The figure shows three views and two pictorial views of one solid part (mm, origin at its lowest corner). Answer the questions. Coordinates: 2 decimals unless noted, no trailing zeros. Order: outer loops, then holes, each group sorted by start corner. A loop starts at its lowest first (then second) coordinate and runs counter-clockwise, first axis right, second up.
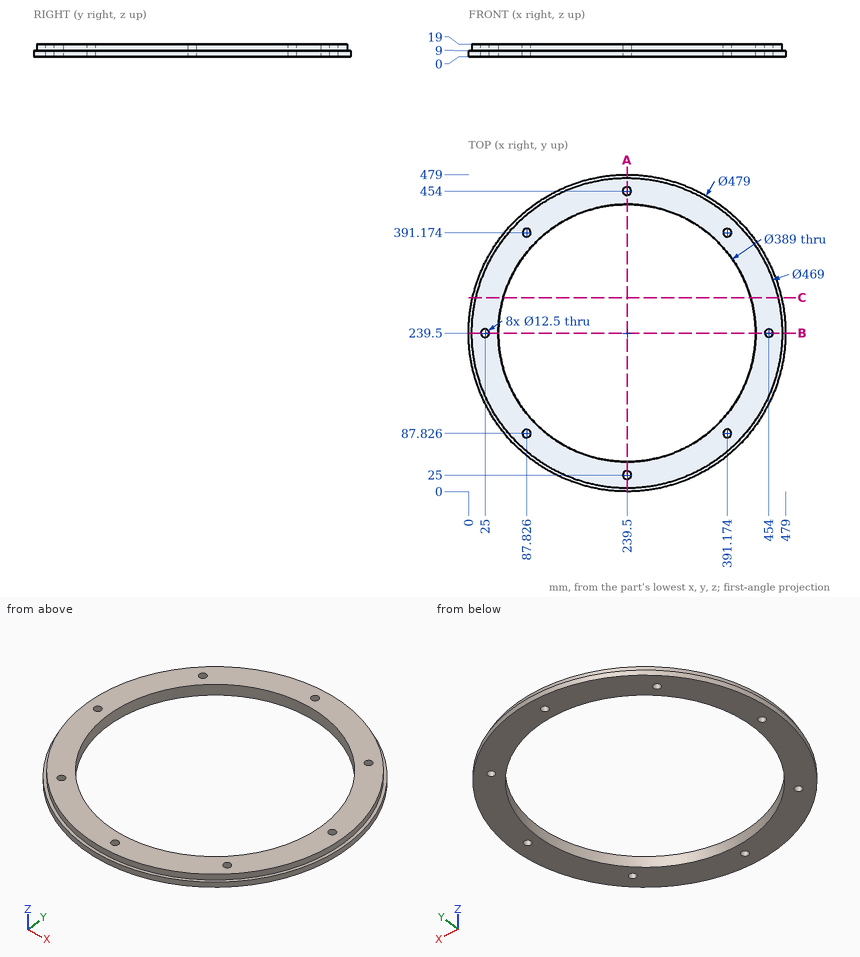
Q1. The part is cut by section C-C, the plane y = 293. Determine the outline of the cut face in (x, z) (1 decimal).
Q2. The part is cut by section A-A, the plane x = 239.5. Determine the outline of the cut face in (y, z), then the cut area to 4 significant figures.
Q3. Each of these flat-tipped pins is pushed along its axis until it touches: P1, Ø5, axis at y = 311, z = 5, coming from the -X side (1 decimal); P2, Ø10, axis at y = 112, z = 2.5, coming from the -X side; P3, Ø3, axis at x = 419, z = 5, coming from the +Y side. Where does it stop, or does it pass through?
Q4. Straight lines are drawn through the part: L1, parallel to Y at x = 239.5, z = 11.5; L2, parallel to Y at x = 239.5, z = 4.75; L3, parallel to X at y = 88.5, z = 13.25 (1 decimal). For each, find the intervals that lie inside material, in ascending order.
Computed values:
1. outline: (6.1, 0) - (52.5, 0) - (52.5, 19) - (11.2, 19) - (11.2, 9) - (6.1, 9) - close; (426.5, 0) - (472.9, 0) - (472.9, 9) - (467.8, 9) - (467.8, 19) - (426.5, 19) - close
2. outline: (0, 0) - (18.75, 0) - (18.75, 19) - (5, 19) - (5, 9) - (0, 9) - close; (31.25, 0) - (45, 0) - (45, 19) - (31.25, 19) - close; (434, 0) - (447.75, 0) - (447.75, 19) - (434, 19) - close; (460.25, 0) - (479, 0) - (479, 9) - (474, 9) - (474, 19) - (460.25, 19) - close
2. area: 1,135 mm2
3. P1: stops at x = 10.2
3. P2: stops at x = 33.7
3. P3: stops at y = 399.74
4. L1: y = 5 to 18.75, 31.25 to 45, 434 to 447.75, 460.25 to 474
4. L2: y = 0 to 18.75, 31.25 to 45, 434 to 447.75, 460.25 to 479
4. L3: x = 60.1 to 81.6, 94 to 116.9, 362.1 to 385, 397.4 to 418.9
